The listing builds one solid part. Answer for the finished solid, in the listing's coordinates (mm). A direction names the side the tool comes from. Round coordinates to 2 decimals unless told otherwise and drop trailing zeros. Order: outer loops, then holes, each group sorted by start corner. A loop starts at its lowest first (then second) coordinate and runs counter-clockwise, first axis right, second up. Notation, with made-up numbers: (43, 17.5) - (47, 17.5) arc R27 cw to (47, 42.5) - close; hole circle Ø8 at (51, 45). An arc over 180 degrees is marked (long way). Use CSV: the item, a comma, the result in double quotes. Start each with the question number.
Item 1: Find section C-C, the plane y = 4.5. Count the separate pieces of the cut face and the enclosed holes in it, plus the area to 3 significant figures.
Item 2: Find section A-A, the plane x = 34.5. Give the vertices of the cut face in (y, z).
Item 3: Flat-ended cylindrical pins translate along their axes: P1, Ø5, axis at x = 42, z = -7, coming from the +Y side; P2, Ø4, axis at x = 15, y = 3.5, coming from the +Z side; P3, Ø0.9, axis at y = 5, z = -20.5, coming from the -X side; P4, Ø1.2, axis at x = 36, z = -2.5, coming from the -Y side. Find the tip coordinate at first contact, or state that the pin passes through.
Item 4: For faces 1 (the flat face through (17.754, 5.563, -23.811)), 2 (the flat face through (19, 1, -1)), 3 (the flat face through (47, 1, -21)), 4 (the flat face through (38.5, 0.5, -20.9)), 5 (the flat face through (40.754, 5.563, -0.811)), determine the directions among +Z, -Z, +X, -X, +Y, -Y from which every point of the face is accessible in a straight line to the end or side of a thin tool.
Item 5: Find section B-B, the plane z = -13.1. Give the vertices of the cut face in (x, y), plus the area to 3 significant figures.
Item 6: Determine the mould class of faces 6 (the flat face through (19, 6, -23)), 7 (the flat face through (30.5, 0.5, -5.4)) for opening direction Z: +Z half, -Z half, draft (parallel to the pull), parting line (faces both ways), or undercut.
Item 7: Straight lines are drawn through the part: line 1 along X through (y, z) = (6.5, -13.1); line 2 along X through (y, z) = (5.25, -22.75); line 3 along Y through (x, z) = (21, -8.25). For each, find the intervals that lie inside material, in ascending order. Write a range as [from, to].
Item 8: Find section D-D, the plane x = 11. Give the vertices of the cut face in (y, z), plus the area to 3 significant figures.
```python
from build123d import *

# Parameters (mm, degrees)
SKETCH1_W           = 47.6
SKETCH1_H           = 24.6
BOSS_EXTRUDE1_DEPTH = 10
SKETCH2_R           = 10.75
CUT_EXTRUDE1_DEPTH  = 9
CUT_EXTRUDE2_DEPTH  = 9
SKETCH5_W           = 1.6
SKETCH5_H           = 24.6
CUT_EXTRUDE3_DEPTH  = 10
SKETCH6_W           = 46
SKETCH6_H           = 1.6
CUT_EXTRUDE4_DEPTH  = 10
BOSS_EXTRUDE2_DEPTH = 9
SKETCH10_W          = 46
SKETCH10_H          = 8.003908937
CUT_EXTRUDE5_DEPTH  = 1
SKETCH11_W          = 8
SKETCH11_H          = 23
CUT_EXTRUDE6_DEPTH  = 1


with BuildPart() as part:
    # Sketch1 → Boss-Extrude1 (new body)
    with BuildSketch(Plane(origin=(0, 0, 0), x_dir=(1, 0, 0), z_dir=(0, 1, 0))):
        with Locations((23.8, 12.3)):
            Rectangle(SKETCH1_W, SKETCH1_H)
    extrude(amount=BOSS_EXTRUDE1_DEPTH)

    # Sketch2 → Cut-Extrude1 (cut)
    with BuildSketch(Plane(origin=(0, 10, 0), x_dir=(1, 0, 0), z_dir=(0, 1, 0))):
        with Locations(Location((11.5, 13.1, 0), (0, 0, 270))):
            Circle(SKETCH2_R)
        with Locations(Location((34.5, 13.1, 0), (0, 0, 270))):
            Circle(SKETCH2_R)
    extrude(amount=-CUT_EXTRUDE1_DEPTH, mode=Mode.SUBTRACT)

    # Sketch3 → Cut-Extrude2 (cut)
    with BuildSketch(Plane(origin=(0, 10, 0), x_dir=(1, 0, 0), z_dir=(0, 1, 0))):
        Polygon((3, 24.6), (2.5, 23), (5.5, 23), (5, 24.6), align=None)
        Polygon((18, 24.6), (17.5, 23), (20.5, 23), (20, 24.6), align=None)
        Polygon((26, 24.6), (25.5, 23), (28.5, 23), (28, 24.6), align=None)
        Polygon((41, 24.6), (40.5, 23), (43.5, 23), (43, 24.6), align=None)
        Polygon((0, 21.6), (1.6, 22.1), (1.6, 19.1), (0, 19.6), align=None)
        Polygon((0, 6.6), (1.6, 7.1), (1.6, 4.1), (0, 4.6), align=None)
    extrude(amount=-CUT_EXTRUDE2_DEPTH, mode=Mode.SUBTRACT)

    # Sketch5 → Cut-Extrude3 (cut)
    with BuildSketch(Plane(origin=(0, 10, 0), x_dir=(1, 0, 0), z_dir=(0, 1, 0))):
        with Locations((46.8, 12.3)):
            Rectangle(SKETCH5_W, SKETCH5_H)
    extrude(amount=-CUT_EXTRUDE3_DEPTH, mode=Mode.SUBTRACT)

    # Sketch6 → Cut-Extrude4 (cut)
    with BuildSketch(Plane(origin=(0, 10, 0), x_dir=(1, 0, 0), z_dir=(0, 1, 0))):
        with Locations((23, 0.8)):
            Rectangle(SKETCH6_W, SKETCH6_H)
    extrude(amount=-CUT_EXTRUDE4_DEPTH, mode=Mode.SUBTRACT)

    # Sketch7 → Boss-Extrude2 (add)
    with BuildSketch(Plane(origin=(0, 10, 0), x_dir=(1, 0, 0), z_dir=(0, 1, 0))):
        Polygon((46, 21.6), (47.6, 22.1), (47.6, 19.1), (46, 19.6), align=None)
        Polygon((46, 6.6), (47.6, 7.1), (47.6, 4.1), (46, 4.6), align=None)
        Polygon((3, 1.6), (2.5, 0), (5.5, 0), (5, 1.6), align=None)
        Polygon((18, 1.6), (17.5, 0), (20.5, 0), (20, 1.6), align=None)
        Polygon((26, 1.6), (25.5, 0), (28.5, 0), (28, 1.6), align=None)
        Polygon((41, 1.6), (40.5, 0), (43.5, 0), (43, 1.6), align=None)
    extrude(amount=-BOSS_EXTRUDE2_DEPTH)

    # Sketch10 → Cut-Extrude5 (cut)
    with BuildSketch(Plane.XZ):
        with Locations((23, -13.101954469)):
            Rectangle(SKETCH10_W, SKETCH10_H)
    extrude(amount=-CUT_EXTRUDE5_DEPTH, mode=Mode.SUBTRACT)

    # Sketch11 → Cut-Extrude6 (cut)
    with BuildSketch(Plane.XZ):
        with Locations((11.5, -13.1)):
            Rectangle(SKETCH11_W, SKETCH11_H)
        with Locations((34.5, -13.1)):
            Rectangle(SKETCH11_W, SKETCH11_H)
    extrude(amount=-CUT_EXTRUDE6_DEPTH, mode=Mode.SUBTRACT)


solid = part.part
```
Worked out:
1,separate pieces,"1"
1,enclosed holes,"2"
1,area,"332 mm²"
2,outline,"(1, -24.6) - (10, -24.6) - (10, -23.85) - (1, -23.85) - close; (1, -2.35) - (10, -2.35) - (10, -1.6) - (1, -1.6) - close"
3,P1,"stops at y = 10"
3,P2,"stops at z = -1.6"
3,P3,"stops at x = 1.6"
3,P4,"stops at y = 1"
4,face 1,"+Y"
4,face 2,"+Z, +X, -X, -Y"
4,face 3,"+Z, -Z, +X, -Y"
4,face 4,"+Z, -Z, -Y"
4,face 5,"+Y, -Y"
5,outline,"(0, 1) - (0.75, 1) - (0.75, 10) - (0, 10) - close; (22.25, 1) - (23.75, 1) - (23.75, 10) - (22.25, 10) - close; (45.25, 1) - (46, 1) - (46, 10) - (45.25, 10) - close"
5,area,"27.0 mm²"
6,face 6,"undercut"
6,face 7,"draft"
7,line 1,"x = [0, 0.75], [22.25, 23.75], [45.25, 46]"
7,line 2,"x = [0, 6.76], [16.24, 29.76], [39.24, 46]"
7,line 3,"y = [0, 1]"
8,outline,"(1, -24.6) - (10, -24.6) - (10, -23.84) - (1, -23.84) - close; (1, -2.36) - (10, -2.36) - (10, -1.6) - (1, -1.6) - close"
8,area,"13.7 mm²"
